from build123d import *

# Parameters (mm, degrees)
SKETCH1_R           = 30
BOSS_EXTRUDE1_DEPTH = 44
BOSS_EXTRUDE2_DEPTH = 12
BOSS_EXTRUDE3_DEPTH = 15
CUT_EXTRUDE1_DEPTH  = 92.983694207
SKETCH5_R           = 6
CUT_EXTRUDE2_DEPTH  = 98.908120194


with BuildPart() as part:
    # Sketch1 → Boss-Extrude1 (new body)
    with BuildSketch(Plane(origin=(0, 0, 0), x_dir=(1, 0, 0), z_dir=(0, 1, 0))):
        with Locations(Location((0, 0, 0), (0, 0, 270))):
            Circle(SKETCH1_R)
    extrude(amount=BOSS_EXTRUDE1_DEPTH)

    # Sketch2 → Boss-Extrude2 (add)
    with BuildSketch(Plane(origin=(0, 0, 0), x_dir=(1, 0, 0), z_dir=(0, 1, 0))):
        with BuildLine():
            Line((50, 8), (75, 8))
            ThreePointArc((75, 8), (73.430488051, 10.198766547), (71.055490967, 11.486140207))
            Line((71.055490967, 11.486140207), (7.99189246, 28.915906607))
            ThreePointArc((7.99189246, 28.915906607), (30, 0), (7.99189246, -28.915906607))
            Line((7.99189246, -28.915906607), (71.055490967, -11.486140207))
            ThreePointArc((71.055490967, -11.486140207), (73.430488051, -10.198766547), (75, -8))
            Line((75, -8), (50, -8))
            ThreePointArc((50, -8), (42, 0), (50, 8))
        make_face()
    extrude(amount=BOSS_EXTRUDE2_DEPTH)

    # Sketch3 → Boss-Extrude3 (add, symmetric)
    with BuildSketch(Plane.XY):
        with BuildLine():
            Line((-36, 36), (-23.901481141, 36))
            Line((-23.901481141, 36), (-23.901481141, 8))
            Line((-23.901481141, 8), (-36, 8))
            ThreePointArc((-36, 8), (-50, 22), (-36, 36))
        make_face()
    extrude(amount=BOSS_EXTRUDE3_DEPTH, both=True)

    # Sketch4 → Cut-Extrude1 (cut, through all)
    with BuildSketch(Plane(origin=(0, 0, 0), x_dir=(1, 0, 0), z_dir=(0, 1, 0))):
        with BuildLine():
            Line((-72.566045066, 0), (-72.566045066, 3))
            Line((-72.566045066, 3), (-18.761663039, 3))
            ThreePointArc((-18.761663039, 3), (19, 0), (-18.761663039, -3))
            Line((-18.761663039, -3), (-72.566045066, -3))
            Line((-72.566045066, -3), (-72.566045066, 0))
        make_face()
    extrude(amount=CUT_EXTRUDE1_DEPTH, mode=Mode.SUBTRACT)

    # Sketch5 → Cut-Extrude2 (cut, through all)
    with BuildSketch(Plane.XY.offset(15)):
        with Locations((-36, 22)):
            Circle(SKETCH5_R)
    extrude(amount=-CUT_EXTRUDE2_DEPTH, mode=Mode.SUBTRACT)


solid = part.part
Could you check a few things on this model? Use its own coordinates, in mm. A direction names the side the tool comes from. Give positions to 0.01 mm unless a question says otherwise; leave off trailing zeros. Order: outer loops, then holes, each group sorted by start corner. A loop starts at its lowest first (then second) coordinate and runs counter-clockwise, first axis right, second up.
Item 1: If we section it at B-B, the plane x = -10.5: Write out the boundary of the cut face in (y, z), plus the area to 3 significant figures.
Item 2: If we section it at D-D, the plane y = 10: Write out the boundary of the cut face in (x, z).
Item 3: If we section it at A-A, the plane y = 22: Write out the boundary of the cut face in (x, z), plus the area to 3 significant figures.
Item 4: If we mould it in two halves opening along Y, with no side actions, what happens to faces 4 (the face through (-42, 22, -9)), 5 (the face through (18.983, 21.692, -0.793)), 6 (the face through (-32, 8, 9))? For each: pulls with the +Y half, pulls with the -Y half, needs draft (parallel to the pull), parting line crosses it, or undercut.
Item 5: If we section it at C-C, the plane z = -10: Write out the boundary of the cut face in (x, y), plus the area to 3 significant figures.
Item 6: I'm going to push flat-ended pins straight in: pin 1 (9.5 mm diameter, centred on x = -36, y = 22, fed in from -Z); pin 2 (6 mm diameter, centred on x = 66.5, y = 8.5, fed in from +Z); pin 3 (1 mm diameter, centred on y = 19, z = -16.5, fed in from -X); pin 4 (25 mm diameter, centred on x = -37.5, y = 12.5, fed in from -Z). Where does each tip first touch, or does it pass through?
Item 7: I need wall thicknesses on line 1 (Z direction, x = 0, y = 28.5); line 2 (Y direction, x = -36, z = 6.25); line 3 (X direction, y = 25.5, z = 5). Which ranges of each line are inside material? Lowest first, please.
Item 8: For faces 1 (the face through (62, 6, -8)), 2 (the face through (-28, 22, -3)), 3 (the face through (-38, 16, -15)), which set-ups out of +Z, -Z, +X, -X, +Y, -Y let a thin tool reach every point of the face, with its end or its side?
Values:
1. outline: (0, -28.1) - (44, -28.1) - (44, -15.84) - (0, -15.84) - close; (0, 15.84) - (44, 15.84) - (44, 28.1) - (0, 28.1) - close
1. area: 1,080 mm2
2. outline: (-43.21, -15) - (-25.98, -15) arc R30 ccw to (7.99, -28.92) - (71.06, -11.49) arc R6 ccw to (75, -8) - (50, -8) arc R8 cw to (50, 8) - (75, 8) arc R6 ccw to (71.06, 11.49) - (7.99, 28.92) arc R30 ccw to (-25.98, 15) - (-43.21, 15) - (-43.21, 3) - (-18.76, 3) arc R19 cw (long way) to (-18.76, -3) - (-43.21, -3) - close
3. outline: (-50, -15) - (-42, -15) - (-42, -3) - (-50, -3) - close; (-50, 3) - (-42, 3) - (-42, 15) - (-50, 15) - close; (-30, -15) - (-25.98, -15) arc R30 ccw (long way) to (-25.98, 15) - (-30, 15) - (-30, 3) - (-18.76, 3) arc R19 cw (long way) to (-18.76, -3) - (-30, -3) - close
3. area: 1,860 mm2
4. face 4: undercut
4. face 5: needs draft
4. face 6: pulls with the -Y half
5. outline: (-36, 8) - (-28.28, 8) - (-28.28, 0) - (-16.16, 0) - (-16.16, 44) - (-28.28, 44) - (-28.28, 36) - (-36, 36) arc R14 ccw to start; (16.16, 0) - (73.64, 0) - (73.64, 12) - (28.28, 12) - (28.28, 44) - (16.16, 44) - close; hole circle Ø12 at (-36, 22)
5. area: 2,020 mm2
6. pin 1: passes through
6. pin 2: stops at z = 13.57
6. pin 3: stops at x = -25.38
6. pin 4: stops at z = -16.58
7. line 1: z = -30 to -19, 19 to 30
7. line 2: y = 8 to 16, 28 to 36
7. line 3: x = -49.56 to -40.87, -31.13 to -18.33, 18.33 to 29.58
8. face 1: +X, +Y, -Y
8. face 2: -X, +Y, -Y
8. face 3: -Z, -X, +Y, -Y
